The figure shows three views and two pictorial views of one solid part (mm, origin at its lowest corner). Answer the questions. Coordinates: 2 decimals unless noted, no trailing zeros. Order: outer loops, then holes, each group sorted by start corner. A loop starts at its lowest first (then second) coordinate and runs counter-clockwise, first axis right, second up. Notation, with made-up numbers: M -14,3 L 37,3 A22 cw 37,35 Z; hole C 37,-34.75 d4. An arc over 180 degrees is marked long. Answer in a Markdown table with one row per item. Add a question column.
Item 1: The part is cut by section A-A (z = 38). Write down the section's boundary in (x, y).
Item 2: The part is cut by section C-C (x = 59). Write down the section's boundary in (y, z).
Item 3: The part is cut by section B-B (y = 0.25). Write down the section's boundary in (x, z) (1 decimal), then the cut area to 3 significant figures.
Item 4: Flat-ended cylindrical pins translate along their axes: pin 1 Ø0.5 at (x, y) = (3, 1) entering from -Z; pin 2 Ø0.5 at (y, z) = (1, 12.5) entering from -X; pin 3 Ø0.5 at (y, z) = (1, 21) entering from +X. Find the tip coordinate at first contact, or state that the pin passes through.
Item 5: Consider line 1 (X direction, y = 1.5, z = 38.5) (1 decimal); line 2 (Z direction, x = 61, y = 1.05); line 3 (X direction, y = 0.2, z = 18) (1 decimal). Determine where each line is inside the solid, lowest interval first. Write a range as from..to.
Item 6: The part is cut by section D-D (z = 12). Write down the section's boundary in (x, y) (1 decimal).
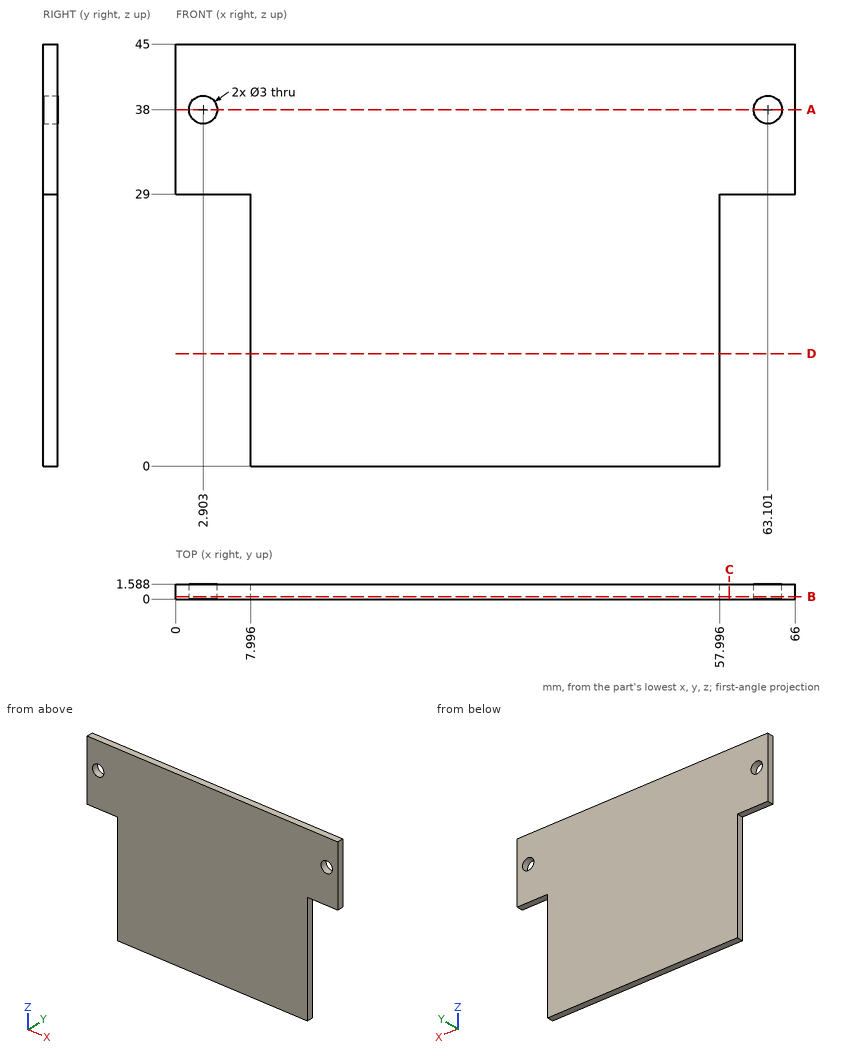
Reply:
| question | item | result |
|---|---|---|
| 1 | outline | M 0,0 L 1.4,0 L 1.4,1.59 L 0,1.59 Z; M 4.4,0 L 61.6,0 L 61.6,1.59 L 4.4,1.59 Z; M 64.6,0 L 66,0 L 66,1.59 L 64.6,1.59 Z |
| 2 | outline | M 0,29 L 1.59,29 L 1.59,45 L 0,45 Z |
| 3 | outline | M 0,29 L 8,29 L 8,0 L 58,0 L 58,29 L 66,29 L 66,45 L 0,45 Z; hole C 2.9,38 d3; hole C 63.1,38 d3 |
| 3 | area | 2,490 mm2 |
| 4 | pin 1 | stops at z = 29 |
| 4 | pin 2 | stops at x = 8 |
| 4 | pin 3 | stops at x = 58 |
| 5 | line 1 | x = 0..1.5, 4.3..61.7, 64.5..66 |
| 5 | line 2 | z = 29..45 |
| 5 | line 3 | x = 8..58 |
| 6 | outline | M 8,0 L 58,0 L 58,1.6 L 8,1.6 Z |
